CAD build for the part. Positions are in the model's coordinates, mm. Face numbers are marked on the shaded views. A direction names the side the tool comes from. Give positions to 0.01 mm unless a question says otherwise; leave off trailing zeros. Order: outer loops, then holes, each group sorted by start corner. A loop starts at its lowest first (then second) coordinate and runs counter-clockwise, first axis right, second up. Notation, with made-up numbers: M 29.5,62.25 L 59.5,62.25 A26 ccw 59.5,85.25 Z; hole C -38.75,74.5 d10. An arc over 180 degrees is marked long. Put each result on its own line as item: value. Start each with the question number.
1) Two-plate mould, pull along Y, no slides. Class the marked faces 6, 7 and 8: released by +Y, released by -Y, zero draft, split by the parting line, or undercut.
2) Pin check, flat tips, straight feed: pin 1 (1.5 mm diameter, centred on y = -2, z = -11, fed in from -X); pin 2 (3 mm diameter, centred on x = 52, z = 12.34, fed in from -Y); pin 3 (1.3 mm diameter, centred on x = 14, y = 2.5, fed in from -Z); pin 4 (1.8 mm diameter, centred on y = 6.5, z = -12, fed in from -X). Stop position of each tip, or through.
3) Cut at B-B (y = 0.75). Give the number of separate pieces and of enclosed holes in the cut face, and give its area (3 significant figures).
4) Cut at A-A (x = 52). Write the cut outline in (y, z), and give its area (3 significant figures).
5) Drill centre lines: line 1 (Y direction, x = 12.5, z = -13); line 2 (Y direction, x = 35, z = 4.5); line 3 (Y direction, x = 30, z = -10). Where is each one in solid material? Low to high. Write a range as [from, to].
6) Cut at C-C (z = -8). Write the cut outline in (x, y).
7) Cut at D-D (y = 5.5). Write the cut outline in (x, z).
8) Tool access for the marked faces 1, 2, 3, 4 and 5: list every direction of +Z, -Z, +X, -X, +Y, -Y with a clear straight run to the whole face (end or side of a thin tool).
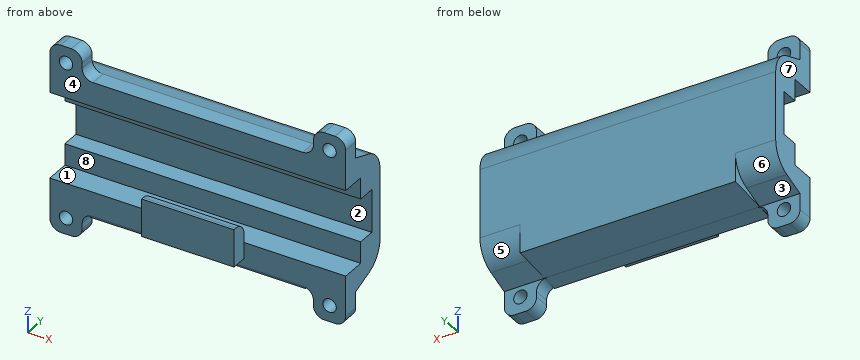
```python
from build123d import *

# Parameters (mm, degrees)
BOSS_EXTRUDE1_DEPTH = 55
FILLET2_R           = 5
SKETCH2_W           = 6
SKETCH2_H           = 5
BOSS_EXTRUDE2_DEPTH = 3
FILLET3_R           = 2
SKETCH3_R           = 1.25
CUT_EXTRUDE1_DEPTH  = 3
SKETCH5_W           = 17.2
SKETCH5_H           = 7
BOSS_EXTRUDE4_DEPTH = 3
BOSS_EXTRUDE5_START = 7.5
BOSS_EXTRUDE5_DEPTH = 40
SKETCH7_W           = 63.002691758
SKETCH7_H           = 45.786839941
CUT_EXTRUDE2_DEPTH  = 10
FILLET5_R           = 2.5


# Read off the part's stored shape, not the designer's step: Boss-Extrude5
with BuildPart() as part:
    # Sketch1 → Boss-Extrude1 (new body)
    with BuildSketch(Plane(origin=(0, 0, 0), x_dir=(0, 0, -1), z_dir=(1, 0, 0))):
        Polygon((10.162208757, 0), (10.162208757, 4.5), (6.162208757, 4.5), (6.162208757, 7.8), (-1.837791243, 7.8), (-1.837791243, 4.5), (-5.837791243, 4.5), (-5.837791243, 0), (-10.337791243, 0), (-10.337791243, 3), (-7.753679525, 10.3), (12.078097038, 10.3), (14.662208757, 3), (14.662208757, 0), align=None)
    extrude(amount=BOSS_EXTRUDE1_DEPTH)

    # Fillet2
    fillet2_edges = [part.edges().sort_by_distance(p)[0] for p in [
        (27.5, 10.3, 7.753679525),
        (27.5, 10.3, -12.078097038),
    ]]
    fillet(fillet2_edges, radius=FILLET2_R)

    # Sketch2 → Boss-Extrude2 (add)
    with BuildSketch(Plane.XZ):
        with Locations((3, 12.837791243)):
            Rectangle(SKETCH2_W, SKETCH2_H)
        with Locations((52, 12.837791243)):
            Rectangle(SKETCH2_W, SKETCH2_H)
        with Locations((52, -17.162208757)):
            Rectangle(SKETCH2_W, SKETCH2_H)
        with Locations((3, -17.162208757)):
            Rectangle(SKETCH2_W, SKETCH2_H)
    extrude(amount=-BOSS_EXTRUDE2_DEPTH)

    # Fillet3
    fillet3_edges = [part.edges().sort_by_distance(p)[0] for p in [
        (0, 1.5, 15.337791243),
        (6, 1.5, 15.337791243),
        (6, 1.5, 10.337791243),
        (55, 1.5, 15.337791243),
        (49, 1.5, 10.337791243),
        (49, 1.5, 15.337791243),
        (55, 1.5, -19.662208757),
        (49, 1.5, -19.662208757),
        (49, 1.5, -14.662208757),
        (0, 1.5, -19.662208757),
        (6, 1.5, -14.662208757),
        (6, 1.5, -19.662208757),
    ]]
    fillet(fillet3_edges, radius=FILLET3_R)

    # Sketch3 → Cut-Extrude1 (cut)
    with BuildSketch(Plane(origin=(0, 3, 0), x_dir=(1, 0, 0), z_dir=(0, 1, 0))):
        with Locations(Location((3, -12.337791243, 0), (0, 0, 270))):
            Circle(SKETCH3_R)
        with Locations(Location((3, 16.662208757, 0), (0, 0, 270))):
            Circle(SKETCH3_R)
        with Locations(Location((52, 16.662208757, 0), (0, 0, 270))):
            Circle(SKETCH3_R)
        with Locations(Location((52, -12.337791243, 0), (0, 0, 270))):
            Circle(SKETCH3_R)
    extrude(amount=-CUT_EXTRUDE1_DEPTH, mode=Mode.SUBTRACT)

    # Sketch5 → Boss-Extrude4 (add)
    with BuildSketch(Plane.XZ):
        with Locations((27.5, -9.662208757)):
            Rectangle(SKETCH5_W, SKETCH5_H)
    extrude(amount=BOSS_EXTRUDE4_DEPTH)

    # Boss-Extrude5 outline → Boss-Extrude5 (add)
    with BuildSketch(Plane.YZ.offset(BOSS_EXTRUDE5_START)):
        with BuildLine():
            Line((6.96848703, -13.257412341), (3, -14.662208757))
            Line((3, -14.662208757), (11.563888282, -13.687484192))
            Line((11.563888282, -13.687484192), (10.3, -2.583015869))
            Line((10.3, -2.583015869), (10.3, -8.544011124))
            ThreePointArc((10.3, -8.544011124), (9.383040237, -11.429974122), (6.96848703, -13.257412341))
        make_face()
        Polygon((0, -14.662208757), (0.038366584, -14.999295924), (3, -14.662208757), align=None)
    extrude(amount=BOSS_EXTRUDE5_DEPTH)

    # Sketch7 → Cut-Extrude2 (cut)
    with BuildSketch(Plane(origin=(0, 10.3, 0), x_dir=(1, 0, 0), z_dir=(0, 1, 0))):
        with Locations((26.50814736, 1.093849158)):
            Rectangle(SKETCH7_W, SKETCH7_H)
    extrude(amount=CUT_EXTRUDE2_DEPTH, mode=Mode.SUBTRACT)

    # Fillet5
    fillet5_edges = [part.edges().sort_by_distance(p)[0] for p in [
        (27.5, 0, -6.162208757),
    ]]
    fillet(fillet5_edges, radius=FILLET5_R)


solid = part.part
```
Solution:
1. face 6: released by +Y
1. face 7: zero draft
1. face 8: undercut
2. pin 1: x = 18.9
2. pin 2: y = 0
2. pin 3: z = -14.79
2. pin 4: x = 0
3. separate pieces: 2
3. enclosed holes: 4
3. area: 602 mm²
4. outline: M 0,-19.66 L 3,-19.66 L 3,-17.91 L 0,-17.91 Z; M 0,-15.41 L 3,-15.41 L 3,-14.66 L 6.97,-13.26 A5 ccw 10.3,-8.54 L 10.3,4.22 A5 ccw 6.97,8.93 L 3,10.34 L 3,11.09 L 0,11.09 L 0,5.84 L 4.5,5.84 L 4.5,1.84 L 7.8,1.84 L 7.8,-6.16 L 4.5,-6.16 L 4.5,-10.16 L 0,-10.16 Z; M 0,13.59 L 3,13.59 L 3,15.34 L 0,15.34 Z
4. area: 151 mm²
5. line 1: [0, 10.3]
5. line 2: [4.5, 10.29]
5. line 3: [-3, 0], [4.5, 10.3]
6. outline: M 0,4.5 L 55,4.5 L 55,10.3 L 0,10.3 Z; M 18.9,-3 L 36.1,-3 L 36.1,-0.09 L 18.9,-0.09 Z
7. outline: M 0,-13.78 L 7.5,-13.78 L 7.5,-14.38 L 47.5,-14.38 L 47.5,-13.78 L 55,-13.78 L 55,-6.16 L 0,-6.16 Z; M 0,1.84 L 55,1.84 L 55,9.45 L 0,9.45 Z
8. face 1: +X, -X
8. face 2: +X, -X, -Y
8. face 3: -Z, -X, +Y
8. face 4: +Z, +X, -X, -Y
8. face 5: -Z, +X, +Y
